Check sheet for the modelled part. Datum: model origin and axes. Units: mm. A direction names the side the tool comes from. Round coordinates to 2 decimals unless told otherwise and drop trailing zeros. Write each loop counter-clockwise with the first axis right and the second up, starting at its lowest first coordinate (ties: lowest second). Pieces come first, ordered by that corner, then holes. Notation, with made-up numbers: (-15.75, -26.75) -> (15.25, -26.75) arc R6 ccw to (15.25, -21.75) -> close; hole circle Ø6 at (-35, 61). An arc over 180 degrees is marked (long way). One line per item, written item: value.
from build123d import *

# Parameters (mm, degrees)
CYLINDER076_R           = 2.5
CYLINDER076_DEPTH       = 27
CYLINDER075_R           = 2.75
CYLINDER075_DEPTH       = 10
BOX033_W                = 10
BOX033_H                = 10
BOX033_DEPTH            = 30
CYLINDER051_R           = 1.6
CYLINDER051_DEPTH       = 28
CYLINDER051_ROLL_ANGLE  = 90
CYLINDER050_R           = 1.6
CYLINDER050_DEPTH       = 28
CYLINDER050_ROLL_ANGLE  = 90
CYLINDER049_R           = 1.6
CYLINDER049_DEPTH       = 28
CYLINDER049_ROLL_ANGLE  = 90
CYLINDER048_R           = 1.6
CYLINDER048_DEPTH       = 28
CYLINDER048_ROLL_ANGLE  = 90
CYLINDER044_R           = 1.6
CYLINDER044_DEPTH       = 28
CYLINDER044_ROLL_ANGLE  = 90
CYLINDER043_R           = 1.6
CYLINDER043_DEPTH       = 28
CYLINDER043_ROLL_ANGLE  = 90
CYLINDER042_R           = 1.6
CYLINDER042_DEPTH       = 28
CYLINDER042_ROLL_ANGLE  = 90
CYLINDER041_R           = 1.6
CYLINDER041_DEPTH       = 28
CYLINDER041_ROLL_ANGLE  = 90
CYLINDER047_R           = 0.85
CYLINDER047_DEPTH       = 10
CYLINDER046_R           = 0.85
CYLINDER046_DEPTH       = 10
BOX025_W                = 22
BOX025_H                = 4
BOX025_DEPTH            = 5
CYLINDER045_R           = 3.25
CYLINDER045_DEPTH       = 10
CYLINDER045_PITCH_ANGLE = 90
BOX024_W                = 55
BOX024_H                = 31
BOX024_DEPTH            = 13
BOX021_W                = 61
BOX021_H                = 34
BOX021_DEPTH            = 13
BOX023_W                = 12
BOX023_H                = 3
BOX023_DEPTH            = 13
BOX022_W                = 12
BOX022_H                = 3
BOX022_DEPTH            = 13


with BuildPart() as cylinder128:
    # Cylinder076 → Cylinder076 (new body)
    with BuildSketch(Plane(origin=(-9, -20, 14), x_dir=(1, 0, 0), z_dir=(0, 0, 1))):
        Circle(CYLINDER076_R)
    extrude(amount=CYLINDER076_DEPTH)


with BuildPart() as obj1:
    # Cylinder075 → Cylinder075 (new body)
    with BuildSketch(Plane(origin=(-9, -20, 4), x_dir=(1, 0, 0), z_dir=(0, 0, 1))):
        Circle(CYLINDER075_R)
    extrude(amount=CYLINDER075_DEPTH)

    # Fusion103: union Cylinder128
    add(cylinder128.part)


with BuildPart() as cut045021:
    # Box033 → Box033 (new body)
    with BuildSketch(Plane(origin=(-14, -25, 9), x_dir=(1, 0, 0), z_dir=(0, 0, 1))):
        with Locations((5, 5)):
            Rectangle(BOX033_W, BOX033_H)
    extrude(amount=BOX033_DEPTH)

    # Cut045021: cut obj1
    add(obj1.part, mode=Mode.SUBTRACT)


with BuildPart() as cylinder103:
    # Cylinder051 → Cylinder051 (new body)
    with BuildSketch(Plane.XY):
        Circle(CYLINDER051_R)
    extrude(amount=CYLINDER051_DEPTH)


with BuildPart() as cylinder103_1:
    # Cylinder051 roll: moved
    add(cylinder103.part.rotate(Axis((0, 0, 0), (1, 0, 0)), CYLINDER051_ROLL_ANGLE))


with BuildPart() as cylinder103_2:
    # Cylinder051 placement: moved
    add(cylinder103_1.part.moved(Location((-23, 20, 36))))


with BuildPart() as fusion085:
    # Cylinder050 → Cylinder050 (new body)
    with BuildSketch(Plane.XY):
        Circle(CYLINDER050_R)
    extrude(amount=CYLINDER050_DEPTH)


with BuildPart() as fusion085_1:
    # Cylinder050 roll: moved
    add(fusion085.part.rotate(Axis((0, 0, 0), (1, 0, 0)), CYLINDER050_ROLL_ANGLE))


with BuildPart() as fusion085_2:
    # Cylinder050 placement: moved
    add(fusion085_1.part.moved(Location((-23, 20, 29))))

    # Fusion085: union Cylinder103
    add(cylinder103_2.part)


with BuildPart() as fusion085_3:
    # Fusion085 placement: moved
    add(fusion085_2.part.moved(Location((-1, 0, 0))))


with BuildPart() as cylinder101:
    # Cylinder049 → Cylinder049 (new body)
    with BuildSketch(Plane.XY):
        Circle(CYLINDER049_R)
    extrude(amount=CYLINDER049_DEPTH)


with BuildPart() as cylinder101_1:
    # Cylinder049 roll: moved
    add(cylinder101.part.rotate(Axis((0, 0, 0), (1, 0, 0)), CYLINDER049_ROLL_ANGLE))


with BuildPart() as cylinder101_2:
    # Cylinder049 placement: moved
    add(cylinder101_1.part.moved(Location((-23, 20, 36))))


with BuildPart() as fusion084:
    # Cylinder048 → Cylinder048 (new body)
    with BuildSketch(Plane.XY):
        Circle(CYLINDER048_R)
    extrude(amount=CYLINDER048_DEPTH)


with BuildPart() as fusion084_1:
    # Cylinder048 roll: moved
    add(fusion084.part.rotate(Axis((0, 0, 0), (1, 0, 0)), CYLINDER048_ROLL_ANGLE))


with BuildPart() as fusion084_2:
    # Cylinder048 placement: moved
    add(fusion084_1.part.moved(Location((-23, 20, 29))))

    # Fusion084: union Cylinder101
    add(cylinder101_2.part)


with BuildPart() as fusion084_3:
    # Fusion084 placement: moved
    add(fusion084_2.part.moved(Location((1, 0, 0))))


with BuildPart() as cylinder096:
    # Cylinder044 → Cylinder044 (new body)
    with BuildSketch(Plane.XY):
        Circle(CYLINDER044_R)
    extrude(amount=CYLINDER044_DEPTH)


with BuildPart() as cylinder096_1:
    # Cylinder044 roll: moved
    add(cylinder096.part.rotate(Axis((0, 0, 0), (1, 0, 0)), CYLINDER044_ROLL_ANGLE))


with BuildPart() as cylinder096_2:
    # Cylinder044 placement: moved
    add(cylinder096_1.part.moved(Location((-23, 20, 36))))


with BuildPart() as fusion080:
    # Cylinder043 → Cylinder043 (new body)
    with BuildSketch(Plane.XY):
        Circle(CYLINDER043_R)
    extrude(amount=CYLINDER043_DEPTH)


with BuildPart() as fusion080_1:
    # Cylinder043 roll: moved
    add(fusion080.part.rotate(Axis((0, 0, 0), (1, 0, 0)), CYLINDER043_ROLL_ANGLE))


with BuildPart() as fusion080_2:
    # Cylinder043 placement: moved
    add(fusion080_1.part.moved(Location((-23, 20, 29))))

    # Fusion080: union Cylinder096
    add(cylinder096_2.part)


with BuildPart() as cylinder094:
    # Cylinder042 → Cylinder042 (new body)
    with BuildSketch(Plane.XY):
        Circle(CYLINDER042_R)
    extrude(amount=CYLINDER042_DEPTH)


with BuildPart() as cylinder094_1:
    # Cylinder042 roll: moved
    add(cylinder094.part.rotate(Axis((0, 0, 0), (1, 0, 0)), CYLINDER042_ROLL_ANGLE))


with BuildPart() as cylinder094_2:
    # Cylinder042 placement: moved
    add(cylinder094_1.part.moved(Location((54, 20, 36))))


with BuildPart() as fusion081:
    # Cylinder041 → Cylinder041 (new body)
    with BuildSketch(Plane.XY):
        Circle(CYLINDER041_R)
    extrude(amount=CYLINDER041_DEPTH)


with BuildPart() as fusion081_1:
    # Cylinder041 roll: moved
    add(fusion081.part.rotate(Axis((0, 0, 0), (1, 0, 0)), CYLINDER041_ROLL_ANGLE))


with BuildPart() as fusion081_2:
    # Cylinder041 placement: moved
    add(fusion081_1.part.moved(Location((54, 20, 29))))

    # Fusion081: union Cylinder094
    add(cylinder094_2.part)


with BuildPart() as cylinder099:
    # Cylinder047 → Cylinder047 (new body)
    with BuildSketch(Plane(origin=(8.35, -29, 40), x_dir=(1, 0, 0), z_dir=(0, 0, -1))):
        Circle(CYLINDER047_R)
    extrude(amount=CYLINDER047_DEPTH)


with BuildPart() as fusion078:
    # Cylinder046 → Cylinder046 (new body)
    with BuildSketch(Plane(origin=(20.65, -29, 30), x_dir=(1, 0, 0), z_dir=(0, 0, 1))):
        Circle(CYLINDER046_R)
    extrude(amount=CYLINDER046_DEPTH)

    # Fusion078: union Cylinder099
    add(cylinder099.part)


with BuildPart() as cut039:
    # Box025 → Box025 (new body)
    with BuildSketch(Plane(origin=(3.5, -31, 34), x_dir=(1, 0, 0), z_dir=(0, 0, 1))):
        with Locations((11, 2)):
            Rectangle(BOX025_W, BOX025_H)
    extrude(amount=BOX025_DEPTH)

    # Cut039: cut Fusion078
    add(fusion078.part, mode=Mode.SUBTRACT)


with BuildPart() as cylinder097:
    # Cylinder045 → Cylinder045 (new body)
    with BuildSketch(Plane.XY):
        Circle(CYLINDER045_R)
    extrude(amount=CYLINDER045_DEPTH)


with BuildPart() as cylinder097_1:
    # Cylinder045 pitch: moved
    add(cylinder097.part.rotate(Axis((0, 0, 0), (0, 1, 0)), CYLINDER045_PITCH_ANGLE))


with BuildPart() as cylinder097_2:
    # Cylinder045 placement: moved
    add(cylinder097_1.part.moved(Location((36, -17.25, 32.5))))


with BuildPart() as cube023:
    # Box024 → Box024 (new body)
    with BuildSketch(Plane(origin=(-13, -24, 26), x_dir=(1, 0, 0), z_dir=(0, 0, 1))):
        with Locations((27.5, 15.5)):
            Rectangle(BOX024_W, BOX024_H)
    extrude(amount=BOX024_DEPTH)


with BuildPart() as fusion079:
    # Box021 → Box021 (new body)
    with BuildSketch(Plane(origin=(-16, -27, 26), x_dir=(1, 0, 0), z_dir=(0, 0, 1))):
        with Locations((30.5, 17)):
            Rectangle(BOX021_W, BOX021_H)
    extrude(amount=BOX021_DEPTH)

    # Cut037: cut Cube023
    add(cube023.part, mode=Mode.SUBTRACT)

    # Cut038: cut Cylinder097
    add(cylinder097_2.part, mode=Mode.SUBTRACT)

    # Fusion079: union Cut039
    add(cut039.part)


with BuildPart() as fusion082:
    # Box023 → Box023 (new body)
    with BuildSketch(Plane(origin=(-28, 4, 26), x_dir=(1, 0, 0), z_dir=(0, 0, 1))):
        with Locations((6, 1.5)):
            Rectangle(BOX023_W, BOX023_H)
    extrude(amount=BOX023_DEPTH)

    # Fusion082: union Fusion079
    add(fusion079.part)


with BuildPart() as obj2:
    # Box022 → Box022 (new body)
    with BuildSketch(Plane(origin=(45, 4, 26), x_dir=(1, 0, 0), z_dir=(0, 0, 1))):
        with Locations((6, 1.5)):
            Rectangle(BOX022_W, BOX022_H)
    extrude(amount=BOX022_DEPTH)

    # Fusion083: union Fusion082
    add(fusion082.part)

    # Cut040: cut Fusion081
    add(fusion081_2.part, mode=Mode.SUBTRACT)

    # Cut041: cut Fusion080
    add(fusion080_2.part, mode=Mode.SUBTRACT)

    # Cut042: cut Fusion084
    add(fusion084_3.part, mode=Mode.SUBTRACT)

    # Cut043: cut Fusion085
    add(fusion085_3.part, mode=Mode.SUBTRACT)

    # Fusion104: union Cut045021
    add(cut045021.part)


solid = obj2.part
Item 1: Mould release check, pull along Z, two halves, no side actions. Record for faces 1 (the flat face through (57, 5, 32)), 2 (the flat face through (14, -29, 34)), 3 (the cylindrical face through (-25.6, 5.5, 29)): pulls with the +Z half, pulls with the -Z half, needs draft (parallel to the pull), parting line crosses it, or undercut.
Answer:
face 1: needs draft
face 2: pulls with the -Z half
face 3: undercut
Item 2: Depth check by flat-ended pin: P1, Ø4, axis at y = -5, z = 30, coming from the +X side; P2, Ø11, axis at x = -7.5, z = 17, coming from the -Y side; P3, Ø9.5, axis at x = 48.5, z = 32, coming from the -Y side. Enter the tip coordinate at first touch or a pass-through.
Answer:
P1: stops at x = 45
P2: stops at y = -25
P3: stops at y = -27
Item 3: Sectioned sample at B-B on x = 20.65. Enter the section's corners in (y, z).
Answer:
outline: (-31, 34) -> (-29.85, 34) -> (-29.85, 39) -> (-31, 39) -> close; (-28.15, 34) -> (-27, 34) -> (-27, 26) -> (-24, 26) -> (-24, 39) -> (-28.15, 39) -> close
Item 4: Sectioned sample at A-A on z = 32.5. Enter the section's corners in (x, y).
Answer:
outline: (-28, 4) -> (-16, 4) -> (-16, -27) -> (45, -27) -> (45, -20.5) -> (42, -20.5) -> (42, -24) -> (-4, -24) -> (-4, -15) -> (-13, -15) -> (-13, 7) -> (-28, 7) -> close; (42, -14) -> (45, -14) -> (45, 4) -> (57, 4) -> (57, 7) -> (42, 7) -> close; hole circle Ø5 at (-9, -20)
Item 5: Sectioned sample at D-D on z = 16. Enter the section's corners in (x, y), and give its area (3 significant figures).
Answer:
outline: (-14, -25) -> (-4, -25) -> (-4, -15) -> (-14, -15) -> close; hole circle Ø5 at (-9, -20)
area: 80.4 mm^2
Item 6: Tool access check on faces 4 (the flat face through (3.5, -29, 36)), 5 (the flat face through (-14, -20, 17)), 6 (the cylindrical face through (43.48, -16.27, 29.4)). Record the directions out of +Z, -Z, +X, -X, +Y, -Y that give a thin tool (end or side, any length) a straight path to the whole face; none if there is none.
Answer:
face 4: +Z, -Z, -X, -Y
face 5: -Z, -X, +Y, -Y
face 6: +X
Item 7: Thickness scan on line 1 (X direction, y = -0.5, z = 34.75); line 2 (X direction, y = -21, z = 28); line 3 (X direction, y = -20, z = 11.05). Record the ranges inside material, lowest first.
Answer:
line 1: x = -16 to -13, 42 to 45
line 2: x = -16 to -11.29, -6.71 to -4, 42 to 45
line 3: x = -14 to -11.75, -6.25 to -4
Item 8: Sectioned sample at C-C on x = 54. Enter the section's corners in (y, z).
Answer:
outline: (4, 26) -> (7, 26) -> (7, 27.4) -> (4, 27.4) -> close; (4, 30.6) -> (7, 30.6) -> (7, 34.4) -> (4, 34.4) -> close; (4, 37.6) -> (7, 37.6) -> (7, 39) -> (4, 39) -> close
